Input: dimensioned drawing with shaded views. Units: mm. Origin: part minimum x, y, z. A direction names the side the tool comes from. Round coordinates to 2 decimals unless told otherwise and drop trailing zeros. Loops run counter-clockwise (first coordinate to the right, second up) from the corner with the lowest first, then second, coordinate; pieces in that order, holes last.
Item 1: Section query D-D on z = 1.5. Return loops of the section in (x, y), then the cut area to 3 significant figures.
Item 2: Access query for the marked faces 4 and 5. Directions: +Z, -Z, +X, -X, +Y, -Y. A direction counts if a zero-diameter tool reaches every point of the face in a straight line with its end or side. Return the directions, or none.
Item 3: First-contact query: P1, Ø4, axis at x = 6.5, y = 7, coming from the +Z side; P2, Ø1.5, axis at x = 5, z = 5.5, coming from the +Y side; P3, Ø2, axis at x = 11, z = 5, coming from the -Y side; P4, Ø5, axis at x = 4, y = 8.5, coming from the -Z side. Flat tips, straight axial feed; report the tip coordinate or a pass-through.
Item 4: Section query A-A on x = 7.5. Return loops of the section in (y, z).
Item 5: Ray query, L1, parallel to Y at x = 7.5, z = 4.3; L2, parallel to Z at x = 8, y = 10.5; L3, parallel to X at y = 8.5, z = 4. Return the intervals inside material, ascending.
Item 6: Pull-direction query (X, two-part tool) for the marked faces 1, 2 and 3; classes: released by +X, released by -X, zero draft, split by the parting line, or undercut.
Item 7: Section query C-C on z = 5. Return loops of the section in (x, y).
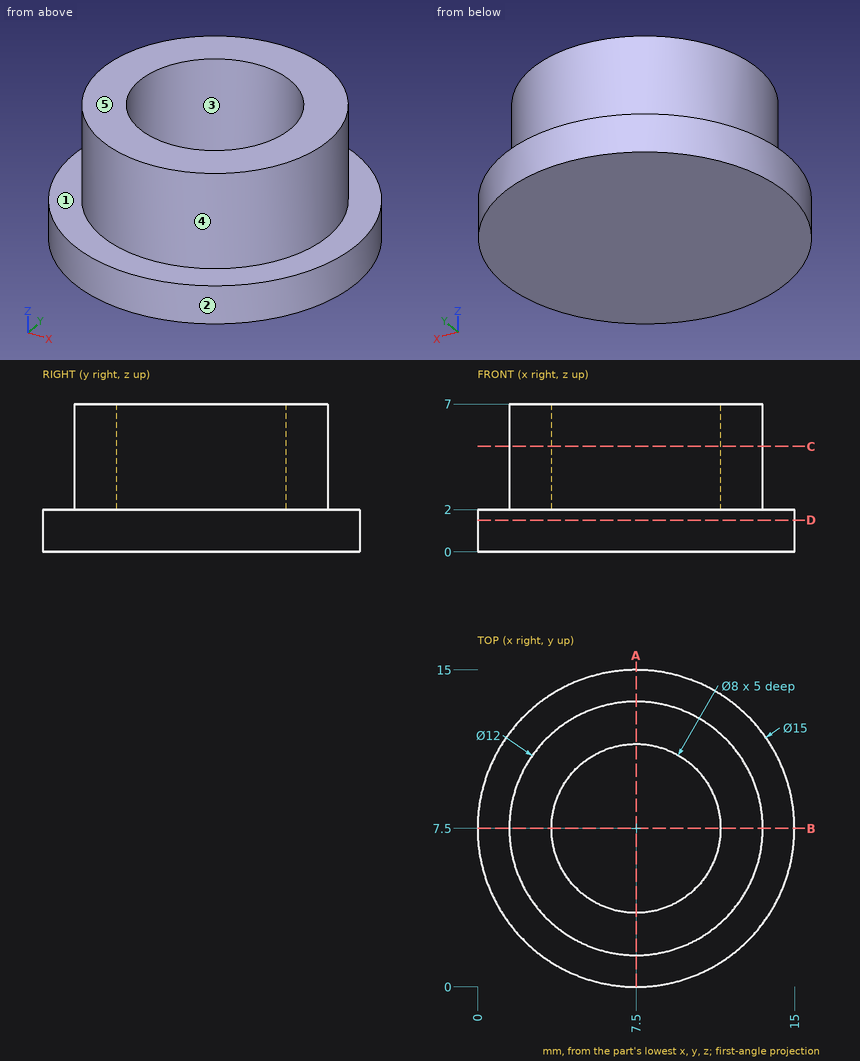
Data:
1. outline: circle Ø15 at (7.5, 7.5)
1. area: 177 mm2
2. face 4: +Z
2. face 5: +Z, +X, -X, +Y, -Y
3. P1: stops at z = 2
3. P2: stops at y = 13.24
3. P3: stops at y = 2.05
3. P4: stops at z = 0
4. outline: (0, 0) - (15, 0) - (15, 2) - (13.5, 2) - (13.5, 7) - (11.5, 7) - (11.5, 2) - (3.5, 2) - (3.5, 7) - (1.5, 7) - (1.5, 2) - (0, 2) - close
5. L1: y = 1.5 to 3.5, 11.5 to 13.5
5. L2: z = 0 to 2
5. L3: x = 1.58 to 3.63, 11.37 to 13.42
6. face 1: zero draft
6. face 2: split by the parting line
6. face 3: undercut
7. outline: circle Ø12 at (7.5, 7.5); hole circle Ø8 at (7.5, 7.5)
